from build123d import *

# Parameters (mm, degrees)
SKETCH1_W           = 24
SKETCH1_H           = 3.8
BOSS_EXTRUDE1_DEPTH = 40
SKETCH2_R           = 1.55
CUT_EXTRUDE1_DEPTH  = 42.933757285
SKETCH3_W           = 30
SKETCH3_H           = 10
BOSS_EXTRUDE2_DEPTH = 20


with BuildPart() as part:
    # Sketch1 → Boss-Extrude1 (new body)
    with BuildSketch(Plane(origin=(0, 0, 0), x_dir=(0, 0, -1), z_dir=(1, 0, 0))):
        Rectangle(SKETCH1_W, SKETCH1_H)
    extrude(amount=BOSS_EXTRUDE1_DEPTH)

    # Sketch2 → Cut-Extrude1 (cut, through all)
    with BuildSketch(Plane.XZ.offset(1.9)):
        with Locations(Location((12, 0, 0), (0, 0, 270))):
            Circle(SKETCH2_R)
        with Locations(Location((31, 0, 0), (0, 0, 270))):
            Circle(SKETCH2_R)
    extrude(amount=-CUT_EXTRUDE1_DEPTH, mode=Mode.SUBTRACT)

    # Sketch3 → Boss-Extrude2 (add)
    with BuildSketch(Plane(origin=(40, 0, 0), x_dir=(0, 0, -1), z_dir=(1, 0, 0))):
        with Locations((0, 0.1)):
            Rectangle(SKETCH3_W, SKETCH3_H)
    extrude(amount=BOSS_EXTRUDE2_DEPTH)


solid = part.part
Could you check a few things on this model? Use its own coordinates, in mm. A direction names the side the tool comes from. Coordinates: 2 decimals unless noted, no trailing zeros. Write each loop counter-clockwise with the first axis right and the second up, starting at its lowest first coordinate (ties: lowest second). Pieces come first, ordered by that corner, then holes. Notation, with made-up numbers: M 21.5,36.5 L 59.5,36.5 A27 cw 59.5,66.5 Z; hole C -26.75,3 d4. An arc over 180 degrees is marked long. One line per question, with ' | ' between items.
1) I need wall thicknesses on probe 1 along X at (y, z) = (-0.1, 0); probe 2 along X at (y, z) = (1.75, 13.75); probe 3 along Z at (x, y) = (16, -0.5). Which ranges of each line are inside material? Lowest first, please. Write a range as [from, to].
Checks:
probe 1: [0, 10.45], [13.55, 29.45], [32.55, 60] | probe 2: [40, 60] | probe 3: [-12, 12]
2) Imagine slicing it at D-D, the plane z = -10. Write out the boundary of the cut face in (x, y), and give its area (3 significant figures).
Checks:
outline: M 0,-1.9 L 40,-1.9 L 40,-4.9 L 60,-4.9 L 60,5.1 L 40,5.1 L 40,1.9 L 0,1.9 Z | area: 352 mm²
3) For faces 1 (the face through (20, 0, 12)), 2 (the face through (20, 1.9, 0)), 3 (the face through (20, 0, -12)), 4 (the face through (20, -1.9, 0)), which set-ups out of +Z, -Z, +X, -X, +Y, -Y let a thin tool reach every point of the face, with its end or its side?
Checks:
face 1: +Z, -X, +Y, -Y | face 2: +Z, -Z, -X, +Y | face 3: -Z, -X, +Y, -Y | face 4: +Z, -Z, -X, -Y
4) Imagine slicing it at B-B, the plane z = 0. Write out the boundary of the cut face in (x, y).
Checks:
outline: M 0,-1.9 L 10.45,-1.9 L 10.45,1.9 L 0,1.9 Z; M 13.55,-1.9 L 29.45,-1.9 L 29.45,1.9 L 13.55,1.9 Z; M 32.55,-1.9 L 40,-1.9 L 40,-4.9 L 60,-4.9 L 60,5.1 L 40,5.1 L 40,1.9 L 32.55,1.9 Z
5) Imagine slicing it at C-C, the plane y = 0.5. Write out the boundary of the cut face in (x, z), and give its area (3 significant figures).
Checks:
outline: M 0,-12 L 40,-12 L 40,-15 L 60,-15 L 60,15 L 40,15 L 40,12 L 0,12 Z; hole C 12,0 d3.1; hole C 31,0 d3.1 | area: 1,540 mm²
6) Imagine slicing it at A-A, the plane x = 31. Write out the boundary of the cut face in (y, z).
Checks:
outline: M -1.9,-12 L 1.9,-12 L 1.9,-1.55 L -1.9,-1.55 Z; M -1.9,1.55 L 1.9,1.55 L 1.9,12 L -1.9,12 Z
7) For pin 1 Ø6 at (x, z) = (18.5, -7.5) entering from -Y; pin 2 Ø3 at (x, y) = (15, -1) entering from -Z; pin 3 Ø5 at (x, y) = (29.5, -0.5) entering from +Z, each with a flat end and sliding along its axis, tell me the tip position at first contact or that it passes through.
Checks:
pin 1: y = -1.9 | pin 2: z = -12 | pin 3: z = 12
